Here's how the part is built. I have some questions about the finished solid (model axes, mm). Face numbers are marked on the shaded views. Coordinates: 2 decimals unless noted, no trailing zeros. Order: outer loops, then holes, each group sorted by start corner. A loop starts at its lowest first (then second) coordinate and runs counter-clockwise, first axis right, second up. Notation, with made-up numbers: (67.5, 13) - (97.5, 13) arc R10 ccw to (97.5, 23) - close; hole circle Ø5 at (81, 1). An arc over 180 degrees is marked (long way). Answer in a Markdown table with one row per item. Add a question column.
Item 1: If I drill on line 1 along Y through (x, z) = (6, 3.75); line 2 along Y through (x, z) = (-8.5, 5.75); line 3 along X through (y, z) = (4, 0.75), over which ranges is the centre line in solid material (lowest first)? Write a range as from..to.
Item 2: I want a section at C-C (y = -14). Please give me the cut outline in (x, z).
Item 3: I want a section at A-A (z = 4.25). Please give me the cut outline in (x, y).
Item 4: Thinking about a two-plate mould opening in Y: for the marked faces 1, 2 and 3, which applies, +Y half, -Y half, draft (parallel to the pull), parting line (faces both ways), or undercut?
Item 5: I want a section at B-B (x = 5). Please give me the cut outline in (y, z).
Item 6: Will these pins go through, and if not, where does the flat tip stop? pin 1 Ø3 at (y, z) = (-26.5, 2.5) entering from -X; pin 2 Ø4 at (y, z) = (-27.5, 3.5) entering from +X.
```python
from build123d import *

# Parameters (mm, degrees)
F1_DEPTH = 7.000011
F2_R     = 11
F3_DEPTH = 7.001011


with BuildPart() as f1:
    # F0 (on Top) → F1 (new body)
    with BuildSketch(Plane.XY):
        with BuildLine():
            ThreePointArc((0, -38.1), (15.570026, -15.570026), (38.1, 0))
            ThreePointArc((38.1, 0), (15.570026, 15.570026), (0, 38.1))
            ThreePointArc((0, 38.1), (-15.570026, 15.570026), (-38.1, 0))
            ThreePointArc((-38.1, 0), (-15.570026, -15.570026), (0, -38.1))
        make_face()
    extrude(amount=F1_DEPTH)

    # F2 (on face) → F3 (cut, through all)
    with BuildSketch(Plane.XY.offset(7.000011)):
        Circle(F2_R)
    extrude(amount=-F3_DEPTH, mode=Mode.SUBTRACT)


solid = f1.part
```
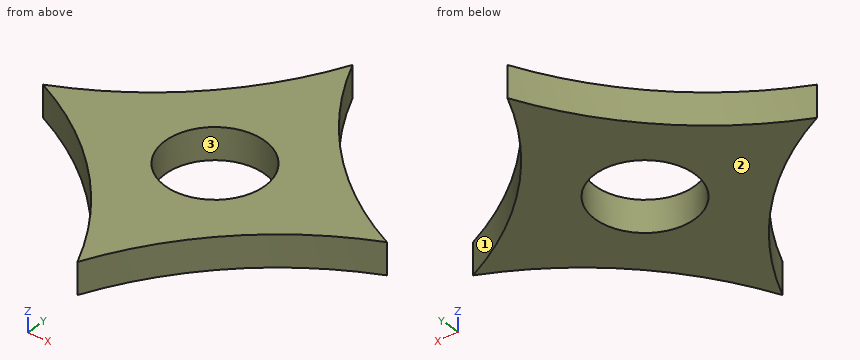
Values follow:
| question | item | result |
|---|---|---|
| 1 | line 1 | y = -27.26..-9.22, 9.22..27.26 |
| 1 | line 2 | y = -23.72..-6.98, 6.98..23.72 |
| 1 | line 3 | x = -30.43..-10.25, 10.25..30.43 |
| 2 | outline | (-17.19, 0) - (17.19, 0) - (17.19, 7) - (-17.19, 7) - close |
| 3 | outline | (-38.1, 0) arc R76.2 cw to (0, -38.1) arc R76.2 cw to (38.1, 0) arc R76.2 cw to (0, 38.1) arc R76.2 cw to start; hole circle Ø22 at (0, 0) |
| 4 | face 1 | +Y half |
| 4 | face 2 | draft |
| 4 | face 3 | undercut |
| 5 | outline | (-28.8, 0) - (-9.8, 0) - (-9.8, 7) - (-28.8, 7) - close; (9.8, 0) - (28.8, 0) - (28.8, 7) - (9.8, 7) - close |
| 6 | pin 1 | stops at x = -7.56 |
| 6 | pin 2 | stops at x = 7.2 |
